For this review, use the dimensioned drawing (mm, ordinates from the lowest corner) and the shaded views. A direction names the side the tool comes from. Round coordinates to 2 decimals unless told otherwise and drop trailing zeros. Write each loop counter-clockwise with the first axis right and the second up, starting at its lowest first coordinate (ties: lowest second). Pieces come first, ordered by that corner, then holes. Notation, with made-up numbers: (-15.75, 56.25) -> (-4.75, 56.25) arc R18 ccw to (-4.75, 75.25) -> close; hole circle Ø7 at (-36, -8). An arc over 180 degrees is marked (long way). Write each question's results on one line, items separated by ' | '. Start each with the question number.
Item 1: Clearance check with flat-ended pins moving along their axes: pin 1 (3 mm diameter, centred on x = 9, y = 6, fed in from +Z); pin 2 (7.5 mm diameter, centred on x = 7.5, y = 16, fed in from +Z); pin 3 (1 mm diameter, centred on x = 9.5, z = 3, fed in from -Y). State where each tip first meets the part, or that it passes through.
Item 2: The part is to be moulded in two halves that separate along Y. For the marked faces 1, 2 and 3, say which applies: +Y half, -Y half, draft (parallel to the pull), parting line (faces both ways), or undercut.
Item 3: Add section D-D (x = 13.25). State the section outline as (y, z) points, plus the area to 4 significant figures.
Item 4: Add section A-A (z = 2). State the section outline as (x, y) points.
Item 5: Add section C-C (y = 15.75). Count the separate pieces of the cut face and the enclosed holes in it, plus the area to 3 significant figures.
Item 6: Tool access review of the marked faces 4 and 5: name each direction out of +Z, -Z, +X, -X, +Y, -Y from which nothing blocks a thin tool from reaching the whole face with its end or side.
Item 7: Add section B-B (x = 7). State the section outline as (y, z) points.
Item 8: To check wall thickness, follow line 1 along Y through (x, z) = (10.5, 2.7); line 2 along Z through (x, y) = (13, 14); line 3 along Y through (x, z) = (7.25, 2.25). State the ranges of each line that lie inside material, in increasing order.
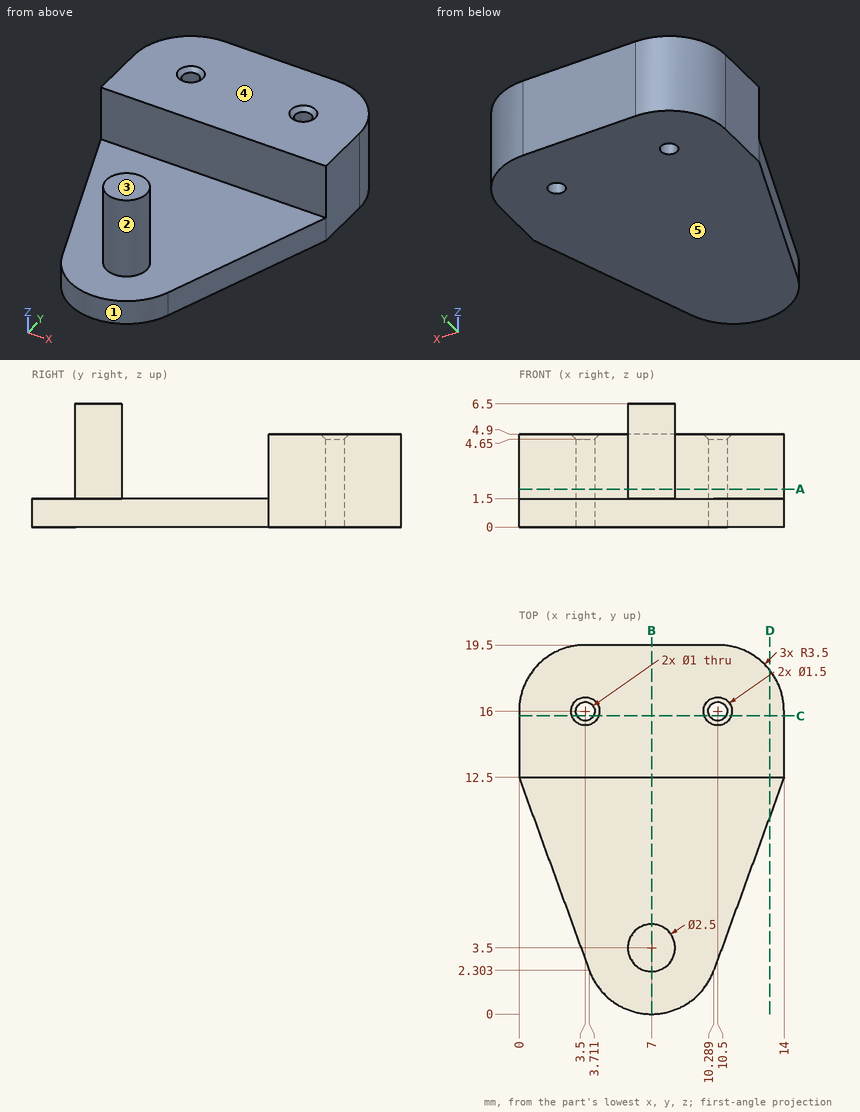
Responses:
1) pin 1: stops at z = 1.5 | pin 2: stops at z = 4.9 | pin 3: stops at y = 12.5
2) face 1: -Y half | face 2: undercut | face 3: draft
3) outline: (10.44, 0) -> (18.17, 0) -> (18.17, 4.9) -> (12.5, 4.9) -> (12.5, 1.5) -> (10.44, 1.5) -> close | area: 30.85 mm^2
4) outline: (0, 12.5) -> (14, 12.5) -> (14, 16) arc R3.5 ccw to (10.5, 19.5) -> (3.5, 19.5) arc R3.5 ccw to (0, 16) -> close; circle Ø2.5 at (7, 3.5); hole circle Ø1 at (3.5, 16); hole circle Ø1 at (10.5, 16)
5) separate pieces: 3 | enclosed holes: 0 | area: 60.0 mm^2
6) face 4: +Z, +X, -X, +Y | face 5: -Z, +X, -X, +Y, -Y
7) outline: (0, 0) -> (19.5, 0) -> (19.5, 4.9) -> (12.5, 4.9) -> (12.5, 1.5) -> (4.75, 1.5) -> (4.75, 6.5) -> (2.25, 6.5) -> (2.25, 1.5) -> (0, 1.5) -> close
8) line 1: y = 12.5 to 15.5, 16.5 to 19.5 | line 2: z = 0 to 4.9 | line 3: y = 2.28 to 4.72, 12.5 to 19.5
